Check sheet for the modelled part. Datum: model origin and axes. Units: mm. Give positions to 0.01 mm unless a question says otherwise; leave off trailing zeros. Order: outer loops, then holes, each group sorted by start corner. A loop starts at its lowest first (then second) coordinate and runs counter-clockwise, first axis right, second up.
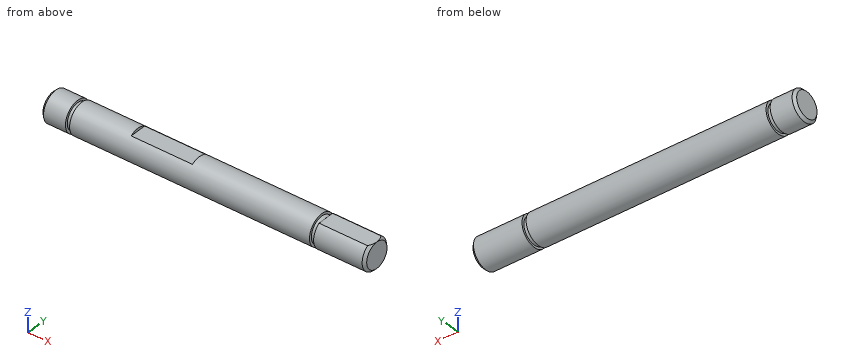
```python
from build123d import *

# Parameters (mm, degrees)
CHAFL_N1_SIZE         = 0.5
CORTAR_EXTRUIR1_START = -10
CORTAR_EXTRUIR1_DEPTH = 10
CORTAR_EXTRUIR2_START = -46.8
CORTAR_EXTRUIR2_DEPTH = 12


with BuildPart() as part:
    # Croquis1 → Revolución1 (revolve)
    with BuildSketch(Plane(origin=(0, 0, 0), x_dir=(-1, 0, 0), z_dir=(0, 1, 0)), mode=Mode.PRIVATE) as revoluci_n1_sk:
        Polygon((-31.7, 0), (-31.7, 3), (-21.7, 3), (-21.7, 2.55), (-20.9, 2.55), (-20.9, 3), (26.1, 3), (26.1, 2.55), (26.9, 2.55), (26.9, 3), (31.7, 3), (31.7, 0), align=None)
    revolve(revoluci_n1_sk.sketch.rotate(Axis((31.7, 0, 0), (-1, 0, 0)), 180), axis=Axis((31.7, 0, 0), (-1, 0, 0)))

    # Chaflán1
    chafl_n1_edges = [part.edges().sort_by_distance(p)[0] for p in [
        (31.7, 0, 3),
        (-31.7, 0, 3),
    ]]
    chamfer(chafl_n1_edges, length=CHAFL_N1_SIZE)

    # Croquis2 → Cortar-Extruir1 (cut)
    with BuildSketch(Plane.YZ.offset(31.7).offset(CORTAR_EXTRUIR1_START)):
        with BuildLine():
            Line((1.658312395, 2.5), (-1.658312395, 2.5))
            ThreePointArc((-1.658312395, 2.5), (0, 3), (1.658312395, 2.5))
        make_face()
    extrude(amount=CORTAR_EXTRUIR1_DEPTH, mode=Mode.SUBTRACT)

    # Croquis2<2> → Cortar-Extruir2 (cut)
    with BuildSketch(Plane.YZ.offset(31.7).offset(CORTAR_EXTRUIR2_START)):
        with BuildLine():
            Line((1.658312395, 2.5), (-1.658312395, 2.5))
            ThreePointArc((-1.658312395, 2.5), (0, 3), (1.658312395, 2.5))
        make_face()
    extrude(amount=CORTAR_EXTRUIR2_DEPTH, mode=Mode.SUBTRACT)


solid = part.part
```
(1) Cross-section at A-A on x = 26. Enter the section's corners in (y, z), then the cut area to 3 significant figures.
Response values:
outline: (-1.66, 2.5) arc R3 ccw (long way) to (1.66, 2.5) - close
area: 27.1 mm2
(2) Gauge pin test, flat ends, axial feed: pin 1 Ø1.5 at (x, y) = (-18.5, -2.5) entering from +Z; pin 2 Ø3.5 at (x, y) = (28, 0) entering from +Z; pin 3 Ø0.6 at (y, z) = (0, 3) entering from -X. Record the tip position at first contact, or that the pin passes through.
Response values:
pin 1: stops at z = 2.44
pin 2: stops at z = 2.5
pin 3: stops at x = -31.5
(3) Cross-section at B-B on x = 15. Enter the section's corners in (y, z), then the cut area to 3 significant figures.
Response values:
outline: circle Ø6 at (0, 0)
area: 28.3 mm2
(4) Material ranges on L1, parallel to X at y = -0.75, z = -2.5; L2, parallel to X at y = 2, z = 1.75; L3, parallel to Z at x = -11.5, y = 1.85, recorded low to high.
Response values:
L1: x = -31.59 to -26.9, -26.1 to 20.9, 21.7 to 31.59
L2: x = -31.54 to -26.9, -26.1 to 20.9, 21.7 to 31.54
L3: z = -2.36 to 2.36
